Build history of the part. All positions in model axes, mm. Round coordinates to 2 decimals unless told otherwise and drop trailing zeros. Loops run counter-clockwise (first coordinate to the right, second up) from the corner with the lowest first, then second, coordinate; pieces in that order, holes last. Notation, with made-up numbers: (-24, 9) - (6, 9) arc R15 ccw to (6, 22) - close; hole circle Ø10 at (77, 54). An arc over 180 degrees is marked (long way). Use one line per item in the form item = value. Start each with the question number.
Q1. Saw through at C-C (z = 3.5). Give the cut face in (x, y).
Q2. Mould opens along X. For faces 1 (the face through (0, 0, 2)), 2 (the face through (6.691, -12.864, 10.628)), 3 (the face through (0, 0, 0)), 4 (the face through (-9.999, -7.667, 10.872)) say: released by +X, released by -X, zero draft, split by the parting line, or undercut.
Q3. Pin check, flat tips, straight feed: pin 1 (8 mm diameter, centred on x = -11, z = 12.5, fed in from -Y); pin 2 (7.5 mm diameter, centred on x = -5.5, y = -2.5, fed in from +Z); pin 3 (1 mm diameter, centred on y = -5.5, z = 16, fed in from -X). Stop position of each tip, or through.
Q4. Drill centre lines: line 1 (Y direction, x = 0, z = 8.5); line 2 (Z direction, x = 8.5, y = 3.75); line 3 (X direction, y = -7, z = 12). Where is each one in solid material? Low to high.
Q5. Saw through at A-A (x = 0). Give the cut face in (y, z), then the cut area to 3 significant figures.
```python
from build123d import *

# Parameters (mm, degrees)
SKETCH_R        = 14.5
PAD_DEPTH       = 20
SKETCH001_R     = 12.6
POCKET_DEPTH    = 18
CHAMFER_SIZE    = 2
CHAMFER001_SIZE = 0.5
FILLET_R        = 0.5


with BuildPart() as part:
    # Sketch → Pad (new body)
    with BuildSketch(Plane.XY):
        Circle(SKETCH_R)
    extrude(amount=PAD_DEPTH)

    # Sketch001 (on Face3 of Pad) → Pocket (cut)
    with BuildSketch(Plane.XY.offset(20)):
        Circle(SKETCH001_R)
    extrude(amount=-POCKET_DEPTH, mode=Mode.SUBTRACT)

    # Chamfer
    chamfer_edges = [part.edges().sort_by_distance(p)[0] for p in [
        (-14.5, 0, 0),
    ]]
    chamfer(chamfer_edges, length=CHAMFER_SIZE)

    # Chamfer001
    chamfer001_edges = [part.edges().sort_by_distance(p)[0] for p in [
        (-12.6, 0, 20),
    ]]
    chamfer(chamfer001_edges, length=CHAMFER001_SIZE)

    # Fillet
    fillet_edges = [part.edges().sort_by_distance(p)[0] for p in [
        (-14.5, 0, 20),
    ]]
    fillet(fillet_edges, radius=FILLET_R)


solid = part.part
```
Report:
q1.outline = circle Ø29 at (0, 0); hole circle Ø25.2 at (0, 0)
q2.face_1 = undercut
q2.face_2 = split by the parting line
q2.face_3 = zero draft
q2.face_4 = undercut
q3.pin_1 = -12.7
q3.pin_2 = 2
q3.pin_3 = -13.61
q4.line_1 = -14.5 to -12.6, 12.6 to 14.5
q4.line_2 = 0 to 2
q4.line_3 = -12.7 to -10.48, 10.48 to 12.7
q5.outline = (-14.5, 2) - (-12.5, 0) - (12.5, 0) - (14.5, 2) - (14.5, 19.5) arc R0.5 ccw to (14, 20) - (13.1, 20) - (12.6, 19.5) - (12.6, 2) - (-12.6, 2) - (-12.6, 19.5) - (-13.1, 20) - (-14, 20) arc R0.5 ccw to (-14.5, 19.5) - close
q5.area = 122 mm²
